Verification items for the finished model (mm, model axes). A direction names the side the tool comes from. Round coordinates to 2 decimals unless told otherwise and drop trailing zeros. Order: outer loops, then holes, each group sorted by start corner. A loop starts at its lowest first (then second) coordinate and runs counter-clockwise, first axis right, second up. Notation, with made-up numbers: (41, 14) -> (88, 14) arc R25 cw to (88, 48) -> close; hole circle Ø7 at (58, 71). An arc over 180 degrees is marked (long way). Put each result on its own line as item: value.
from build123d import *

# Parameters (mm, degrees)
SKETCH_1_W          = 70
SKETCH_1_H          = 52
EXTRUDE_1_DEPTH     = 3
SKETCH_2_R          = 1.6
SKETCH_2_W          = 24
SKETCH_2_H          = 6
SKETCH_2_W_2        = 11
SKETCH_2_H_2        = 3
CUT_EXTRUDE_1_DEPTH = 4
FILLET_1_R          = 1


with BuildPart() as part:
    # 草图1 → 凸台-拉伸1 (new body)
    with BuildSketch(Plane(origin=(0, 0, 0), x_dir=(1, 0, 0), z_dir=(0, 1, 0))):
        Rectangle(SKETCH_1_W, SKETCH_1_H)
    extrude(amount=EXTRUDE_1_DEPTH)

    # 草图2 → 切除-拉伸1 (cut, through all)
    with BuildSketch(Plane(origin=(0, 3, 0), x_dir=(1, 0, 0), z_dir=(0, 1, 0))):
        with Locations((-21, 9.25)):
            Circle(SKETCH_2_R)
        with Locations((21, 18.25)):
            Circle(SKETCH_2_R)
        with Locations((21, -18.25)):
            Circle(SKETCH_2_R)
        with Locations((0, 26)):
            Rectangle(SKETCH_2_W, SKETCH_2_H)
        with Locations((-29.5, 24.5)):
            Rectangle(SKETCH_2_W_2, SKETCH_2_H_2)
        with Locations((29.5, 24.5)):
            Rectangle(SKETCH_2_W_2, SKETCH_2_H_2)
        with Locations((-29.5, -24.5)):
            Rectangle(SKETCH_2_W_2, SKETCH_2_H_2)
        with Locations((29.5, -24.5)):
            Rectangle(SKETCH_2_W_2, SKETCH_2_H_2)
        with Locations((0, -26)):
            Rectangle(SKETCH_2_W, SKETCH_2_H)
    extrude(amount=-CUT_EXTRUDE_1_DEPTH, mode=Mode.SUBTRACT)

    # 圆角1
    fillet_1_edges = [part.edges().sort_by_distance(p)[0] for p in [
        (12, 1.5, -26),
        (-12, 1.5, -26),
        (-35, 1.5, -23),
        (-24, 1.5, -26),
        (35, 1.5, -23),
        (24, 1.5, -26),
        (-35, 1.5, 23),
        (-24, 1.5, 26),
        (35, 1.5, 23),
        (24, 1.5, 26),
        (-12, 1.5, 26),
        (12, 1.5, 26),
    ]]
    fillet(fillet_1_edges, radius=FILLET_1_R)


solid = part.part
Item 1: Section check D-D on y = 1.65. State how many separate pieces and enclosed holes the cut face has, then the cut area to 3 significant figures.
Check sheet entries:
separate pieces: 1
enclosed holes: 3
area: 3,340 mm^2
Item 2: Release check for a two-part mould opening along Z. For faces 4 (the flat face through (-24, 2, 24)), 5 (the cylindrical face through (20.792, 1.521, 16.664)), 6 (the flat face through (0, 2, 23)) record: +Z half, -Z half, draft (parallel to the pull), parting line (faces both ways), or undercut.
Check sheet entries:
face 4: draft
face 5: undercut
face 6: +Z half
Item 3: Gauge pin test, flat ends, axial feed: pin 1 Ø1 at (y, z) = (2, -24) entering from +X; pin 2 Ø1.5 at (x, y) = (27.5, 2) entering from +Z; pin 3 Ø0.6 at (y, z) = (1, -24.5) entering from -X. Record the tip position at first contact, or that the pin passes through.
Check sheet entries:
pin 1: stops at x = 24
pin 2: stops at z = 23
pin 3: stops at x = -24
Item 4: Section check C-C on x = -21. Record the boundary of the cut face in (y, z), then the cut area to 3 significant figures.
Check sheet entries:
outline: (0, -26) -> (3, -26) -> (3, -10.85) -> (0, -10.85) -> close; (0, -7.65) -> (3, -7.65) -> (3, 26) -> (0, 26) -> close
area: 146 mm^2
Item 5: Tool access check on faces 1 (the flat face through (29, 2, 23)), 2 (the flat face through (24, 2, -24)), 3 (the flat face through (12, 2, -24)). Record the directions out of +Z, -Z, +X, -X, +Y, -Y that give a thin tool (end or side, any length) a straight path to the whole face; none if there is none.
Check sheet entries:
face 1: +Z, +X, +Y, -Y
face 2: -Z, +X, +Y, -Y
face 3: -Z, +Y, -Y
Item 6: Section check B-B on x = 21. Record the boundary of the cut face in (y, z).
Check sheet entries:
outline: (0, -26) -> (3, -26) -> (3, -19.85) -> (0, -19.85) -> close; (0, -16.65) -> (3, -16.65) -> (3, 16.65) -> (0, 16.65) -> close; (0, 19.85) -> (3, 19.85) -> (3, 26) -> (0, 26) -> close
Item 7: Section check A-A on z = -9.25. Record the boundary of the cut face in (x, y).
Check sheet entries:
outline: (-35, 0) -> (-22.6, 0) -> (-22.6, 3) -> (-35, 3) -> close; (-19.4, 0) -> (35, 0) -> (35, 3) -> (-19.4, 3) -> close
Item 8: Material ranges on L1, parallel to Z at x = 21, y = 2; L2, parallel to Z at x = 20, y = 1.3; L3, parallel to X at y = 1.25, z = -9.25, recorded low to high. Write a range as [from, to].
Check sheet entries:
L1: z = [-26, -19.85], [-16.65, 16.65], [19.85, 26]
L2: z = [-26, -19.5], [-17, 17], [19.5, 26]
L3: x = [-35, -22.6], [-19.4, 35]
